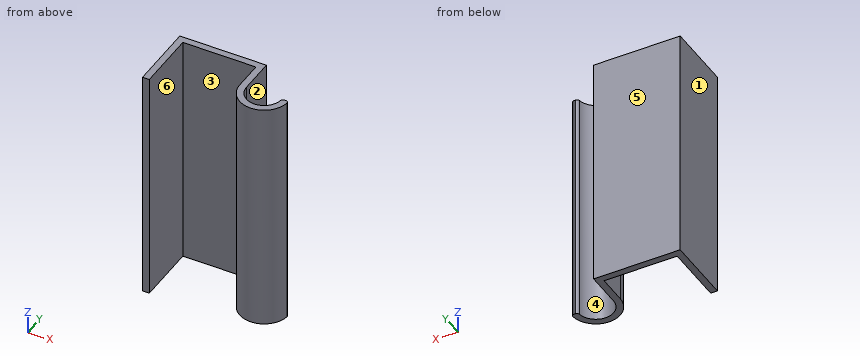
from build123d import *

# Parameters (mm, degrees)
F1_DEPTH = 177.8
F2_R     = 2


with BuildPart() as f1:
    # F0 (on Top) → F1 (new body)
    with BuildSketch(Plane.XY):
        with BuildLine():
            Line((-5.08, 0), (0, 0))
            Line((0, 0), (0, 45.72))
            Line((0, 45.72), (55, 45.72))
            Line((55, 45.72), (55, 23.612564))
            ThreePointArc((55, 23.612564), (73.429315, 5.183249), (91.858629, 23.612564))
            Line((91.858629, 23.612564), (86.778629, 23.612564))
            ThreePointArc((86.778629, 23.612564), (73.429315, 10.263249), (60.08, 23.612564))
            Line((60.08, 23.612564), (60.08, 50.8))
            Line((60.08, 50.8), (-5.08, 50.8))
            Line((-5.08, 50.8), (-5.08, 0))
        make_face()
    extrude(amount=F1_DEPTH)

    # F2
    f2_edges = [f1.edges().sort_by_distance(p)[0] for p in [
        (86.778629, 23.612564, 88.9),
        (91.858629, 23.612564, 88.9),
    ]]
    fillet(f2_edges, radius=F2_R)


solid = f1.part
Source: CAD feature listing. Evaluate the final solid. Frame: model axes, mm. Face numbers are marked on the shaded views. A direction names the side the tool comes from. Round coordinates to 2 decimals unless told otherwise and drop trailing zeros. Loops run counter-clockwise (first coordinate to the right, second up) from the corner with the lowest first, then second, coordinate; pieces in that order, holes last.
Q1. Access query for the marked faces 5 and 6. Directions: +Z, -Z, +X, -X, +Y, -Y. A direction counts if a zero-diameter tool reaches every point of the face in a straight line with its end or side. Return the directions, or none.
Q2. Section D-D, the plane x = 30. Return loops of the section in (y, z).
Q3. First-contact query: P1, Ø10, axis at x = 43, y = 45.5, coming from the -Z side; P2, Ø16.5, axis at x = 24, z = 117, coming from the -Y side; P3, Ø13.5, axis at y = 43, z = 119.5, coming from the +X side; P4, Ø1.2, axis at x = 89, z = 104, coming from the +Y side. Flat tips, straight axial feed; report the tip coordinate or a pass-through.
Q4. Section B-B, the plane z = 45.5. Return loops of the section in (x, y).
Q5. Ray query, line 1 (X direction, y = 44, z = 18.5); line 2 (X direction, y = 15, z = 24); line 3 (Y direction, x = 43, z = 70). Return the intervals inside material, ascending.
Q6. Mould query, pull axis X, two halves, no side actions, for the marked faces 1, 2, 3 and 4. Classes: pulls with the +X half, pulls with the -X half, needs draft (parallel to the pull), parting line crosses it, or undercut.
Q7. Section A-A, the plane y = 35. Return loops of the section in (x, z).
Q8. Section C-C, the plane y = 13. Return loops of the section in (x, z), plus the area to 3 significant figures.
Solutions:
1. face 5: +Z, -Z, +X, -X, +Y
1. face 6: +Z, -Z, -Y
2. outline: (45.72, 0) - (50.8, 0) - (50.8, 177.8) - (45.72, 177.8) - close
3. P1: stops at z = 0
3. P2: stops at y = 45.72
3. P3: stops at x = 60.08
3. P4: stops at y = 23.61
4. outline: (-5.08, 0) - (0, 0) - (0, 45.72) - (55, 45.72) - (55, 23.61) arc R18.43 ccw to (91.72, 21.37) arc R2 ccw to (89.74, 23.61) - (88.65, 23.61) arc R2 ccw to (86.66, 21.87) arc R13.35 cw to (60.08, 23.61) - (60.08, 50.8) - (-5.08, 50.8) - close
5. line 1: x = -5.08 to 0, 55 to 60.08
5. line 2: x = -5.08 to 0, 57.14 to 63.23, 83.63 to 89.72
5. line 3: y = 45.72 to 50.8
6. face 1: pulls with the -X half
6. face 2: pulls with the +X half
6. face 3: undercut
6. face 4: undercut
7. outline: (-5.08, 0) - (0, 0) - (0, 177.8) - (-5.08, 177.8) - close; (55, 0) - (60.08, 0) - (60.08, 177.8) - (55, 177.8) - close
8. outline: (-5.08, 0) - (0, 0) - (0, 177.8) - (-5.08, 177.8) - close; (58.36, 0) - (65.33, 0) - (65.33, 177.8) - (58.36, 177.8) - close; (81.53, 0) - (88.5, 0) - (88.5, 177.8) - (81.53, 177.8) - close
8. area: 3,380 mm2
